Could you check a few things on this model? Use its own coordinates, in mm. A direction names the side the tool comes from. Give positions to 0.01 mm unless a question says otherwise; leave off trailing zeros. Loops run counter-clockwise (first coordinate to the right, second up) from the corner with the lowest first, then second, coordinate; pieces in that order, holes last.
1. Imagine slicing it at B-B (x = 10). List the corners of the cut face in (y, z) for me, plus the area to 3 significant figures.
2. Imagine slicing it at D-D (x = 40). List the corners of the cut face in (y, z) for me, plus the area to 3 significant figures.
3. I need wall thicknesses on line 1 along Y through (x, z) = (55, 3.6); line 2 along X through (y, z) = (-77, 1.7); line 3 along Y through (x, z) = (34, 4.75). Which ranges of each line are inside material? Lowest first, please.
4. For P1, Ø1.8, axis at x = 10, y = -77, coming from the -Z side; P2, Ø4, axis at x = 55, y = -13, coming from the -Z side; P3, Ø9.5, axis at x = 55, y = -77, coming from the +Z side; P4, Ø1.2, axis at y = -22.5, z = 7.5, coming from the +X side, each with a flat end and sliding along its axis, tell me the tip position at first contact or that it passes through.
5. For faces 1 (the flat face through (65, -46, 2)), 2 (the flat face through (3, -44, 5)), 3 (the flat face through (32, -90, 3)), 4 (the cylindrical face through (52, -13, 1)), 5 (the flat face through (32, -3, 5)), which set-ups out of +Z, -Z, +X, -X, +Y, -Y let a thin tool reach every point of the face, with its end or its side?
6. Imagine slicing it at C-C (y = -68.5). List the corners of the cut face in (x, z) for me.
7. Imagine slicing it at A-A (y = -13). List the corners of the cut face in (x, z) for me, plus the area to 3 significant figures.
8. Thinking about a two-plate mould opening in Y: for faces 6 (the flat face through (32, 0, 3)), 7 (the flat face through (32, -44, 0)), 8 (the flat face through (32, -42.5, 5)), which applies, +Y half, -Y half, draft (parallel to the pull), parting line (faces both ways), or undercut?
```python
from build123d import *

# Parameters (mm, degrees)
SKETCH_W        = 65
SKETCH_H        = 90
SKETCH_R        = 1.5
PAD_DEPTH       = 5
SKETCH002_W     = 25
SKETCH002_H     = 90
PAD001_DEPTH    = 4
SKETCH003_W     = 19
SKETCH003_H     = 39.5
POCKET_DEPTH    = 9.001
FILLET_R        = 1
FILLET001_R     = 1
FILLET002_R     = 1
FILLET003_R     = 1
SKETCH004_R     = 3
POCKET001_DEPTH = 3
SKETCH005_W     = 13
SKETCH005_H     = 44
POCKET002_DEPTH = 9.001
FILLET004_R     = 1
FILLET005_R     = 1
FILLET006_R     = 1
FILLET007_R     = 1


with BuildPart() as part:
    # Sketch → Pad (new body)
    with BuildSketch(Plane.XY):
        with Locations((32.5, -45)):
            Rectangle(SKETCH_W, SKETCH_H)
        with Locations((10, -13)):
            Circle(SKETCH_R, mode=Mode.SUBTRACT)
        with Locations((10, -77)):
            Circle(SKETCH_R, mode=Mode.SUBTRACT)
        with Locations((55, -13)):
            Circle(SKETCH_R, mode=Mode.SUBTRACT)
        with Locations((55, -77)):
            Circle(SKETCH_R, mode=Mode.SUBTRACT)
    extrude(amount=PAD_DEPTH)

    # Sketch002 → Pad001 (new body)
    with BuildSketch(Plane.XY.offset(5)):
        with Locations((32.5, -45)):
            Rectangle(SKETCH002_W, SKETCH002_H)
    extrude(amount=PAD001_DEPTH)

    # Sketch003 → Pocket (cut, through all)
    with BuildSketch(Plane.XY.offset(9)):
        with Locations((32.5, -22.75)):
            Rectangle(SKETCH003_W, SKETCH003_H)
        with Locations((32.5, -67.25)):
            Rectangle(SKETCH003_W, SKETCH003_H)
    extrude(amount=-POCKET_DEPTH, mode=Mode.SUBTRACT)

    # Fillet
    fillet_edges = [part.edges().sort_by_distance(p)[0] for p in [
        (23, -47.5, 4.5),
        (23, -3, 4.5),
    ]]
    fillet(fillet_edges, radius=FILLET_R)

    # Fillet001
    fillet001_edges = [part.edges().sort_by_distance(p)[0] for p in [
        (42, -3, 4.5),
        (42, -47.5, 4.5),
    ]]
    fillet(fillet001_edges, radius=FILLET001_R)

    # Fillet002
    fillet002_edges = [part.edges().sort_by_distance(p)[0] for p in [
        (42, -42.5, 4.5),
        (42, -87, 4.5),
    ]]
    fillet(fillet002_edges, radius=FILLET002_R)

    # Fillet003
    fillet003_edges = [part.edges().sort_by_distance(p)[0] for p in [
        (23, -42.5, 4.5),
        (23, -87, 4.5),
    ]]
    fillet(fillet003_edges, radius=FILLET003_R)

    # Sketch004 → Pocket001 (cut)
    with BuildSketch(Plane(origin=(0, 0, 0), x_dir=(1, 0, 0), z_dir=(0, 0, -1))):
        with Locations((10, 77)):
            Circle(SKETCH004_R)
        with Locations((55, 77)):
            Circle(SKETCH004_R)
        with Locations((55, 13)):
            Circle(SKETCH004_R)
        with Locations((10, 13)):
            Circle(SKETCH004_R)
    extrude(amount=-POCKET001_DEPTH, mode=Mode.SUBTRACT)

    # Sketch005 → Pocket002 (cut, through all)
    with BuildSketch(Plane(origin=(0, 0, 0), x_dir=(1, 0, 0), z_dir=(0, 0, -1))):
        with Locations((11.5, 45)):
            Rectangle(SKETCH005_W, SKETCH005_H)
        with Locations((53.5, 45)):
            Rectangle(SKETCH005_W, SKETCH005_H)
    extrude(amount=-POCKET002_DEPTH, mode=Mode.SUBTRACT)

    # Fillet004
    fillet004_edges = [part.edges().sort_by_distance(p)[0] for p in [
        (5, -23, 2.5),
        (47, -23, 2.5),
    ]]
    fillet(fillet004_edges, radius=FILLET004_R)

    # Fillet005
    fillet005_edges = [part.edges().sort_by_distance(p)[0] for p in [
        (5, -67, 2.5),
        (47, -67, 2.5),
    ]]
    fillet(fillet005_edges, radius=FILLET005_R)

    # Fillet006
    fillet006_edges = [part.edges().sort_by_distance(p)[0] for p in [
        (18, -67, 2.5),
        (60, -67, 2.5),
    ]]
    fillet(fillet006_edges, radius=FILLET006_R)

    # Fillet007
    fillet007_edges = [part.edges().sort_by_distance(p)[0] for p in [
        (18, -23, 2.5),
        (60, -23, 2.5),
    ]]
    fillet(fillet007_edges, radius=FILLET007_R)


solid = part.part
```
Derived:
1. outline: (-90, 0) - (-80, 0) - (-80, 3) - (-78.5, 3) - (-78.5, 5) - (-90, 5) - close; (-75.5, 3) - (-74, 3) - (-74, 0) - (-67, 0) - (-67, 5) - (-75.5, 5) - close; (-23, 0) - (-16, 0) - (-16, 3) - (-14.5, 3) - (-14.5, 5) - (-23, 5) - close; (-11.5, 3) - (-10, 3) - (-10, 0) - (0, 0) - (0, 5) - (-11.5, 5) - close
1. area: 182 mm2
2. outline: (-90, 0) - (-87, 0) - (-87, 9) - (-90, 9) - close; (-47.5, 0) - (-42.5, 0) - (-42.5, 9) - (-47.5, 9) - close; (-3, 0) - (0, 0) - (0, 9) - (-3, 9) - close
2. area: 99.0 mm2
3. line 1: y = -90 to -78.5, -75.5 to -67, -23 to -14.5, -11.5 to 0
3. line 2: x = 0 to 7, 13 to 23, 42 to 52, 58 to 65
3. line 3: y = -90 to -87, -47.5 to -42.5, -3 to 0
4. P1: passes through
4. P2: stops at z = 3
4. P3: stops at z = 5
4. P4: stops at x = 45
5. face 1: +Z, -Z, +X, +Y, -Y
5. face 2: +Z, -X, +Y, -Y
5. face 3: +Z, -Z, +X, -X, -Y
5. face 4: -Z
5. face 5: +Z, -Z
6. outline: (0, 0) - (23, 0) - (23, 9) - (20, 9) - (20, 5) - (0, 5) - close; (42, 0) - (65, 0) - (65, 5) - (45, 5) - (45, 9) - (42, 9) - close
7. outline: (0, 0) - (7, 0) - (7, 3) - (8.5, 3) - (8.5, 5) - (0, 5) - close; (11.5, 3) - (13, 3) - (13, 0) - (23, 0) - (23, 9) - (20, 9) - (20, 5) - (11.5, 5) - close; (42, 0) - (52, 0) - (52, 3) - (53.5, 3) - (53.5, 5) - (45, 5) - (45, 9) - (42, 9) - close; (56.5, 3) - (58, 3) - (58, 0) - (65, 0) - (65, 5) - (56.5, 5) - close
7. area: 206 mm2
8. face 6: +Y half
8. face 7: draft
8. face 8: undercut
